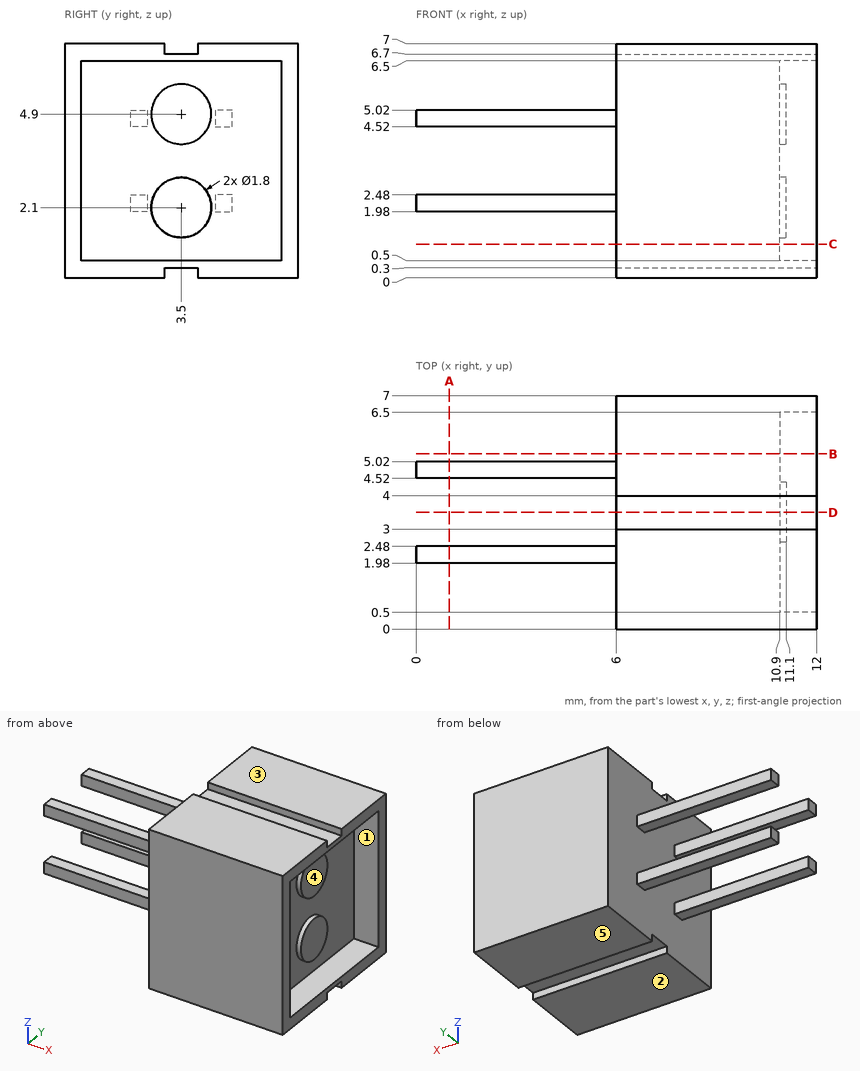
Check sheet for the drawn part. Datum: minimum x, y, z corner. Units: mm. A direction names the side the tool comes from. Give positions to 0.01 mm unless a question says otherwise; leave off trailing zeros. Order: outer loops, then holes, each group sorted by start corner. A loop starts at its lowest first (then second) coordinate and runs counter-clockwise, first axis right, second up. Notation, with made-up numbers: (58, 56.5) - (116, 56.5) arc R12 cw to (116, 67.5) - close; hole circle Ø7 at (45, 83). An arc over 180 degrees is marked (long way). Answer in a Markdown table with one row per item. Add a question column.
Q1. Gauge pin test, flat ends, axial feed: pin 1 (0.6 mm diameter, centred on x = 3.5, z = 4.5, fed in from -Y); pin 2 (0.6 mm diameter, centred on x = 2, z = 5, fed in from +Y); pin 3 (0.5 mm diameter, centred on y = 4, z = 5, fed in from +X). Record the tip position at first contact, or that the pin passes through.
Q2. Material ranges on probe 1 along X at (y, z) = (6.25, 5); probe 2 along X at (y, z) = (5.25, 6.75), recorded low to high. Write a range as from..to.
Q3. Tool access check on the marked faces 4 and 5. Record the directions out of +Z, -Z, +X, -X, +Y, -Y that give a thin tool (end or side, any length) a straight path to the whole face; none if there is none.
Q4. Cross-section at D-D, the plane y = 3.5. Enter the section's corners in (x, z), then the cut area to 3 significant figures.
Q5. Mould release check, pull along Z, two halves, no side actions. Record for the marked faces 1, 2 and 3: pulls with the +Z half, pulls with the -Z half, needs draft (parallel to the pull), parting line crosses it, or undercut.
Q6. Cross-section at A-A, the plane x = 1. Enter the section's corners in (y, z).
Q7. Cross-section at B-B, the plane y = 5.25. Enter the section's corners in (x, z), then the cut area to 3 significant figures.
Check values:
| question | item | result |
|---|---|---|
| 1 | pin 1 | stops at y = 1.98 |
| 1 | pin 2 | stops at y = 5.02 |
| 1 | pin 3 | stops at x = 11.1 |
| 2 | probe 1 | x = 6..10.9 |
| 2 | probe 2 | x = 6..12 |
| 3 | face 4 | +X |
| 3 | face 5 | -Z, +X, -X, +Y, -Y |
| 4 | outline | (6, 0.3) - (12, 0.3) - (12, 0.5) - (10.9, 0.5) - (10.9, 1.2) - (11.1, 1.2) - (11.1, 3) - (10.9, 3) - (10.9, 4) - (11.1, 4) - (11.1, 5.8) - (10.9, 5.8) - (10.9, 6.5) - (12, 6.5) - (12, 6.7) - (6, 6.7) - close |
| 4 | area | 32.5 mm^2 |
| 5 | face 1 | undercut |
| 5 | face 2 | pulls with the -Z half |
| 5 | face 3 | pulls with the +Z half |
| 6 | outline | (1.98, 1.98) - (2.48, 1.98) - (2.48, 2.48) - (1.98, 2.48) - close; (1.98, 4.52) - (2.48, 4.52) - (2.48, 5.02) - (1.98, 5.02) - close; (4.52, 1.98) - (5.02, 1.98) - (5.02, 2.48) - (4.52, 2.48) - close; (4.52, 4.52) - (5.02, 4.52) - (5.02, 5.02) - (4.52, 5.02) - close |
| 7 | outline | (6, 0) - (12, 0) - (12, 0.5) - (10.9, 0.5) - (10.9, 6.5) - (12, 6.5) - (12, 7) - (6, 7) - close |
| 7 | area | 35.4 mm^2 |
